Verification items for the finished model (mm, model axes). A direction names the side the tool comes from. Coordinates: 2 decimals unless noted, no trailing zeros. Loops run counter-clockwise (first coordinate to the right, second up) from the corner with the lowest first, then second, coordinate; pieces in that order, holes last. Notation, with made-up numbers: (73, -29.5) - (132, -29.5) arc R20 cw to (132, 1.5) - close; hole circle Ø3 at (-12, 46). An arc over 180 degrees is marked (long way). One line per item, written item: value. Start each with the question number.
(1) Section check A-A (y = 17). Record the boundary of the cut face in (x, z), plus the area to 3 significant figures.
(2) Section check B-B (x = 5). Record the boundary of the cut face in (y, z), plus the area to 3 significant figures.
(3) Draft check along Y on faces 3 (the face through (3.526, 9.352, -0.986)), 4 (the face through (4.93, 56.4, -0.57)), 5 (the face through (10, 56, -25)), 6 (the face through (5, 55, -25)). Enter one of: +Y half, -Y half, draft (parallel to the pull), parting line (faces both ways), or undercut.
(4) Thickness scan on probe 1 along Z at (x, y) = (1.25, 13); probe 2 along Y at (x, z) = (0.75, -9); probe 3 along Y at (x, z) = (5, -48.55). Record the ranges inside material, lowest first. Write a range as [from, to].
(5) Section check D-D (x = 9.25). Record the boundary of the cut face in (y, z).
(6) Set-up check for faces 1 (the face through (5, 57, -25)), 2 (the face through (5, 27, -2)): record each of +Z, -Z, +X, -X, +Y, -Y from which the full face is reachable in a straight line by a thin tool's end or side.
(7) Gauge pin test, flat ends, axial feed: P1, Ø6, axis at x = 3.5, y = 43, coming from the +Z side; P2, Ø3, axis at x = 4.5, z = -20, coming from the -Y side. Record the tip position at first contact, or that the pin passes through.
(8) Section check C-C (y = 8). Record the boundary of the cut face in (x, z).
```python
from build123d import *

# Parameters (mm, degrees)
EXTRUDE_1_DEPTH     = 10
SKETCH_2_R          = 2
CUT_EXTRUDE_1_DEPTH = 77.47875522


with BuildPart() as part:
    # 草图1 → 凸台-拉伸1 (new body)
    with BuildSketch(Plane(origin=(0, 0, 0), x_dir=(0, 0, -1), z_dir=(1, 0, 0))):
        with BuildLine():
            Line((0, 0), (0, 55))
            ThreePointArc((0, 55), (0.585786438, 56.414213562), (2, 57))
            Line((2, 57), (48, 57))
            ThreePointArc((48, 57), (49.414213562, 56.414213562), (50, 55))
            Line((50, 55), (50, 0))
            Line((50, 0), (48, 0))
            Line((48, 0), (48, 53))
            ThreePointArc((48, 53), (47.414213562, 54.414213562), (46, 55))
            Line((46, 55), (4, 55))
            ThreePointArc((4, 55), (2.585786438, 54.414213562), (2, 53))
            Line((2, 53), (2, 0))
            Line((2, 0), (0, 0))
        make_face()
    extrude(amount=EXTRUDE_1_DEPTH)

    # 草图2 → 切除-拉伸1 (cut, through all)
    with BuildSketch(Plane.XY):
        with Locations((5, 8)):
            Circle(SKETCH_2_R)
    extrude(amount=-CUT_EXTRUDE_1_DEPTH, mode=Mode.SUBTRACT)


solid = part.part
```
Responses:
1. outline: (0, -50) - (10, -50) - (10, -48) - (0, -48) - close; (0, -2) - (10, -2) - (10, 0) - (0, 0) - close
1. area: 40.0 mm²
2. outline: (0, -50) - (6, -50) - (6, -48) - (0, -48) - close; (0, -2) - (6, -2) - (6, 0) - (0, 0) - close; (10, -50) - (55, -50) arc R2 ccw to (57, -48) - (57, -2) arc R2 ccw to (55, 0) - (10, 0) - (10, -2) - (53, -2) arc R2 cw to (55, -4) - (55, -46) arc R2 cw to (53, -48) - (10, -48) - close
2. area: 304 mm²
3. face 3: undercut
3. face 4: +Y half
3. face 5: draft
3. face 6: -Y half
4. probe 1: z = [-50, -48], [-2, 0]
4. probe 2: y = [55, 57]
4. probe 3: y = [0, 6], [10, 56.92]
5. outline: (0, -50) - (55, -50) arc R2 ccw to (57, -48) - (57, -2) arc R2 ccw to (55, 0) - (0, 0) - (0, -2) - (53, -2) arc R2 cw to (55, -4) - (55, -46) arc R2 cw to (53, -48) - (0, -48) - close
6. face 1: +Z, -Z, +X, -X, +Y
6. face 2: +X, -X, -Y
7. P1: stops at z = 0
7. P2: stops at y = 55
8. outline: (0, -50) - (3, -50) - (3, -48) - (0, -48) - close; (0, -2) - (3, -2) - (3, 0) - (0, 0) - close; (7, -50) - (10, -50) - (10, -48) - (7, -48) - close; (7, -2) - (10, -2) - (10, 0) - (7, 0) - close
